from build123d import *

# Parameters (mm, degrees)
F1_DEPTH = 4
F2_SIZE  = 0.8


with BuildPart() as f1:
    # F0 (on Top) → F1 (new body)
    with BuildSketch(Plane.XY):
        with BuildLine():
            Line((9, 6.5), (-9, 6.5))
            ThreePointArc((-9, 6.5), (-11.12132, 5.62132), (-12, 3.5))
            Line((-12, 3.5), (-12, 1))
            ThreePointArc((-12, 1), (-11, 0), (-12, -1))
            Line((-12, -1), (-12, -3.5))
            ThreePointArc((-12, -3.5), (-11.12132, -5.62132), (-9, -6.5))
            Line((-9, -6.5), (9, -6.5))
            ThreePointArc((9, -6.5), (11.12132, -5.62132), (12, -3.5))
            Line((12, -3.5), (12, -1))
            ThreePointArc((12, -1), (11, 0), (12, 1))
            Line((12, 1), (12, 3.5))
            ThreePointArc((12, 3.5), (11.12132, 5.62132), (9, 6.5))
        make_face()
        with BuildLine():
            ThreePointArc((-9, 1.5), (-8.707107, 2.207107), (-8, 2.5))
            Line((-8, 2.5), (-3.5, 2.5))
            ThreePointArc((-3.5, 2.5), (-2.792893, 2.207107), (-2.5, 1.5))
            Line((-2.5, 1.5), (-2.5, -1.5))
            ThreePointArc((-2.5, -1.5), (-2.792893, -2.207107), (-3.5, -2.5))
            Line((-3.5, -2.5), (-8, -2.5))
            ThreePointArc((-8, -2.5), (-8.707107, -2.207107), (-9, -1.5))
            Line((-9, -1.5), (-9, 1.5))
        make_face(mode=Mode.SUBTRACT)
        with BuildLine():
            Line((8, -2.5), (3.5, -2.5))
            ThreePointArc((3.5, -2.5), (2.792893, -2.207107), (2.5, -1.5))
            Line((2.5, -1.5), (2.5, 1.5))
            ThreePointArc((2.5, 1.5), (2.792893, 2.207107), (3.5, 2.5))
            Line((3.5, 2.5), (8, 2.5))
            ThreePointArc((8, 2.5), (8.707107, 2.207107), (9, 1.5))
            Line((9, 1.5), (9, -1.5))
            ThreePointArc((9, -1.5), (8.707107, -2.207107), (8, -2.5))
        make_face(mode=Mode.SUBTRACT)
    extrude(amount=F1_DEPTH)

    # F2
    f2_edges = [f1.edges().sort_by_distance(p)[0] for p in [
        (0, 6.5, 4),
        (-11.12132, 5.62132, 4),
        (-12, 2.25, 4),
        (-11, 0, 4),
        (-12, -2.25, 4),
        (-11.12132, -5.62132, 4),
        (0, -6.5, 4),
        (11.12132, -5.62132, 4),
        (12, -2.25, 4),
        (11, 0, 4),
        (12, 2.25, 4),
        (11.12132, 5.62132, 4),
        (-8.707107, -2.207107, 4),
        (-9, 0, 4),
        (-8.707107, 2.207107, 4),
        (-5.75, 2.5, 4),
        (-2.792893, 2.207107, 4),
        (-2.5, 0, 4),
        (-2.792893, -2.207107, 4),
        (-5.75, -2.5, 4),
        (5.75, -2.5, 4),
        (2.792893, -2.207107, 4),
        (2.5, 0, 4),
        (2.792893, 2.207107, 4),
        (5.75, 2.5, 4),
        (8.707107, 2.207107, 4),
        (9, 0, 4),
        (8.707107, -2.207107, 4),
        (0, 6.5, 0),
        (-11.12132, 5.62132, 0),
        (-12, 2.25, 0),
        (-11, 0, 0),
        (-12, -2.25, 0),
        (-11.12132, -5.62132, 0),
        (0, -6.5, 0),
        (11.12132, -5.62132, 0),
        (12, -2.25, 0),
        (11, 0, 0),
        (12, 2.25, 0),
        (11.12132, 5.62132, 0),
        (-8.707107, -2.207107, 0),
        (-9, 0, 0),
        (-8.707107, 2.207107, 0),
        (-5.75, 2.5, 0),
        (-2.792893, 2.207107, 0),
        (-2.5, 0, 0),
        (-2.792893, -2.207107, 0),
        (-5.75, -2.5, 0),
        (5.75, -2.5, 0),
        (2.792893, -2.207107, 0),
        (2.5, 0, 0),
        (2.792893, 2.207107, 0),
        (5.75, 2.5, 0),
        (8.707107, 2.207107, 0),
        (9, 0, 0),
        (8.707107, -2.207107, 0),
    ]]
    chamfer(f2_edges, length=F2_SIZE)


solid = f1.part
Here's how the part is built. I have some questions about the finished solid (model axes, mm). A direction names the side the tool comes from. Give positions to 0.01 mm unless a question says otherwise; leave off trailing zeros. Order: outer loops, then holes, each group sorted by start corner. A loop starts at its lowest first (then second) coordinate and runs counter-clockwise, first axis right, second up. Notation, with made-up numbers: (57, -22.5) -> (97, -22.5) arc R28 ccw to (97, 12.5) -> close; hole circle Ø11 at (13.25, -25.75). An arc over 180 degrees is marked (long way). One line per item, written item: value. Start each with the question number.
1. We'd pull the mould along Y, two halves only. Please class faces 5 (the face through (0, 0, 0)), 6 (the face through (-2.785, -2.199, 1.983)), 7 (the face through (-10.752, 5.291, 3.694)): released by +Y, released by -Y, zero draft, split by the parting line, or undercut.
2. For faces 1 (the face through (6, 2.5, 2)), 2 (the face through (8.941, -2.421, 3.517)), 3 (the face through (5.7, 2.9, 0.4)), 4 (the face through (-10.8, 0, 3.4)), which set-ups out of +Z, -Z, +X, -X, +Y, -Y let a thin tool reach every point of the face, with its end or its side?
3. Imagine slicing it at B-B, the plane x = 5. List the corners of the cut face in (y, z) for me.
4. Will this pin go through, and if not, where does the flat tip stop? pin 1 Ø1.5 at (y, z) = (5, 1.5) entering from -X.
5. Imagine slicing it at C-C, the plane y = 0. List the corners of the cut face in (x, z) for me, plus the area to 3 significant figures.
6. Imagine slicing it at D-D, the plane z = 3.45. List the corners of the cut face in (x, y) for me, plus the area to 3 significant figures.
7. Imagine slicing it at A-A, the plane z = 1.7. List the corners of the cut face in (x, y) for me, plus the area to 3 significant figures.
8. I need wall thicknesses on probe 1 along Y at (x, z) = (6, 1.7); probe 2 along X at (y, z) = (-2, 2.9); probe 3 along X at (y, z) = (2, 3.45). Which ranges of each line are inside material? Lowest first, please. Write a range as from..to.
Values follow:
1. face 5: zero draft
1. face 6: undercut
1. face 7: released by +Y
2. face 1: +Z, -Z
2. face 2: +Z
2. face 3: -Z
2. face 4: +Z, -X
3. outline: (-6.5, 0.8) -> (-5.7, 0) -> (-3.3, 0) -> (-2.5, 0.8) -> (-2.5, 3.2) -> (-3.3, 4) -> (-5.7, 4) -> (-6.5, 3.2) -> close; (2.5, 0.8) -> (3.3, 0) -> (5.7, 0) -> (6.5, 0.8) -> (6.5, 3.2) -> (5.7, 4) -> (3.3, 4) -> (2.5, 3.2) -> close
4. pin 1: stops at x = -11.9
5. outline: (-11, 0.8) -> (-10.2, 0) -> (-9.8, 0) -> (-9, 0.8) -> (-9, 3.2) -> (-9.8, 4) -> (-10.2, 4) -> (-11, 3.2) -> close; (-2.5, 0.8) -> (-1.7, 0) -> (1.7, 0) -> (2.5, 0.8) -> (2.5, 3.2) -> (1.7, 4) -> (-1.7, 4) -> (-2.5, 3.2) -> close; (9, 0.8) -> (9.8, 0) -> (10.2, 0) -> (11, 0.8) -> (11, 3.2) -> (10.2, 4) -> (9.8, 4) -> (9, 3.2) -> close
5. area: 32.2 mm2
6. outline: (-11.75, -3.5) arc R2.75 ccw to (-9, -6.25) -> (9, -6.25) arc R2.75 ccw to (11.75, -3.5) -> (11.75, -1.22) arc R1.25 cw to (11.75, 1.22) -> (11.75, 3.5) arc R2.75 ccw to (9, 6.25) -> (-9, 6.25) arc R2.75 ccw to (-11.75, 3.5) -> (-11.75, 1.22) arc R1.25 cw to (-11.75, -1.22) -> close; hole (-9.25, -1.5) arc R1.25 ccw to (-8, -2.75) -> (-3.5, -2.75) arc R1.25 ccw to (-2.25, -1.5) -> (-2.25, 1.5) arc R1.25 ccw to (-3.5, 2.75) -> (-8, 2.75) arc R1.25 ccw to (-9.25, 1.5) -> close; hole (2.25, -1.5) arc R1.25 ccw to (3.5, -2.75) -> (8, -2.75) arc R1.25 ccw to (9.25, -1.5) -> (9.25, 1.5) arc R1.25 ccw to (8, 2.75) -> (3.5, 2.75) arc R1.25 ccw to (2.25, 1.5) -> close
6. area: 209 mm2
7. outline: (-12, -3.5) arc R3 ccw to (-9, -6.5) -> (9, -6.5) arc R3 ccw to (12, -3.5) -> (12, -1) arc R1 cw to (12, 1) -> (12, 3.5) arc R3 ccw to (9, 6.5) -> (-9, 6.5) arc R3 ccw to (-12, 3.5) -> (-12, 1) arc R1 cw to (-12, -1) -> close; hole (-9, -1.5) arc R1 ccw to (-8, -2.5) -> (-3.5, -2.5) arc R1 ccw to (-2.5, -1.5) -> (-2.5, 1.5) arc R1 ccw to (-3.5, 2.5) -> (-8, 2.5) arc R1 ccw to (-9, 1.5) -> close; hole (2.5, -1.5) arc R1 ccw to (3.5, -2.5) -> (8, -2.5) arc R1 ccw to (9, -1.5) -> (9, 1.5) arc R1 ccw to (8, 2.5) -> (3.5, 2.5) arc R1 ccw to (2.5, 1.5) -> close
7. area: 238 mm2
8. probe 1: y = -6.5..-2.5, 2.5..6.5
8. probe 2: x = -12..-8.87, -2.63..2.63, 8.87..12
8. probe 3: x = -11.75..-9.15, -2.35..2.35, 9.15..11.75
